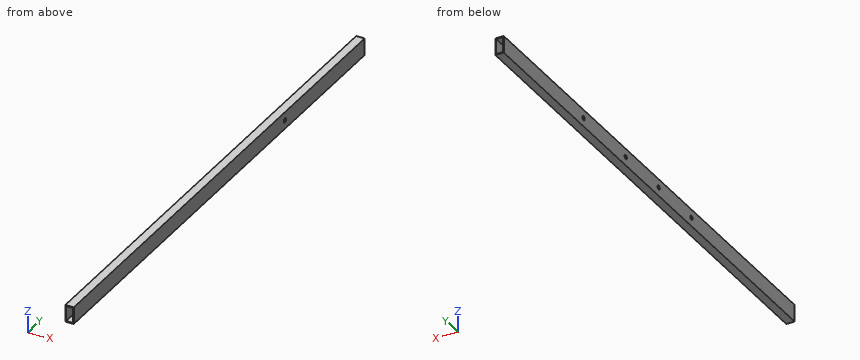
```python
from build123d import *

# Parameters (mm, degrees)
SKETCH_1_W          = 20
SKETCH_1_H          = 40
SKETCH_1_W_2        = 16
SKETCH_1_H_2        = 36
EXTRUDE_1_DEPTH     = 1240
SKETCH_2_R          = 5
CUT_EXTRUDE_1_DEPTH = 21
SKETCH_3_R          = 5
CUT_EXTRUDE_2_DEPTH = 10


with BuildPart() as part:
    # Эскиз1 → Вытянуть-Тонкостенный1 (new body)
    with BuildSketch(Plane(origin=(0, 0, 0), x_dir=(1, 0, 0), z_dir=(0, 1, 0))):
        Rectangle(SKETCH_1_W, SKETCH_1_H)
        Rectangle(SKETCH_1_W_2, SKETCH_1_H_2, mode=Mode.SUBTRACT)
    extrude(amount=EXTRUDE_1_DEPTH)

    # Эскиз2 → Вырез-Вытянуть1 (cut, through all)
    with BuildSketch(Plane(origin=(10, 0, 0), x_dir=(0, 0, -1), z_dir=(1, 0, 0))):
        with Locations((0, 900)):
            Circle(SKETCH_2_R)
    extrude(amount=-CUT_EXTRUDE_1_DEPTH, mode=Mode.SUBTRACT)

    # Эскиз3 → Вырез-Вытянуть2 (cut)
    with BuildSketch(Plane.ZY.offset(10)):
        with Locations((0, 720)):
            Circle(SKETCH_3_R)
        with Locations((0, 580)):
            Circle(SKETCH_3_R)
        with Locations((0, 440)):
            Circle(SKETCH_3_R)
    extrude(amount=-CUT_EXTRUDE_2_DEPTH, mode=Mode.SUBTRACT)


solid = part.part
```
Model file for the job. Use its own axes, mm. Coordinates: 2 decimals unless noted, no trailing zeros. Write each loop counter-clockwise with the first axis right and the second up, starting at its lowest first coordinate (ties: lowest second). Pieces come first, ordered by that corner, then holes. Notation, with made-up numbers: (-22, 37) - (-8, 37) arc R28 cw to (-8, 69) - close; hole circle Ø10 at (-39, -17.75). An arc over 180 degrees is marked (long way). One line per item, written item: value. Start each with the question number.
1. Flat gauge pins, fed straight in: pin 1 (10 mm diameter, centred on x = -1.5, z = 11.5, fed in from +Y); pin 2 (9 mm diameter, centred on y = 580, z = 0, fed in from -X). Where does each tip first touch, or does it go through?
2. Slice it at B-B (z = 11). Write the cut outline in (x, y).
3. Probe line 1 (Y direction, x = -9.15, z = 0); line 2 (X direction, y = 1060, z = 10.5); line 3 (Z direction, x = -5.5, y = 343). List the from-to ranges inside material, lowest first. Write a range as from..to.
4. Slice it at A-A (y = 257). Write the cut outline in (x, z), plus the area to 3 significant figures.
Answers below:
1. pin 1: passes through
1. pin 2: stops at x = 8
2. outline: (-10, 0) - (-8, 0) - (-8, 1240) - (-10, 1240) - close; (8, 0) - (10, 0) - (10, 1240) - (8, 1240) - close
3. line 1: y = 0..435, 445..575, 585..715, 725..895, 905..1240
3. line 2: x = -10..-8, 8..10
3. line 3: z = -20..-18, 18..20
4. outline: (-10, -20) - (10, -20) - (10, 20) - (-10, 20) - close; hole (-8, -18) - (8, -18) - (8, 18) - (-8, 18) - close
4. area: 224 mm^2
